Answer from the drawing. Dimensions are ordinates in mm from the lowest x, y and z of the part. Give positions to 0.01 mm unless a question says otherwise; leave off trailing zeros. Order: outer loops, then holes, each group sorted by start corner. A loop starts at its lowest first (then second) coordinate and runs counter-clockwise, first axis right, second up.
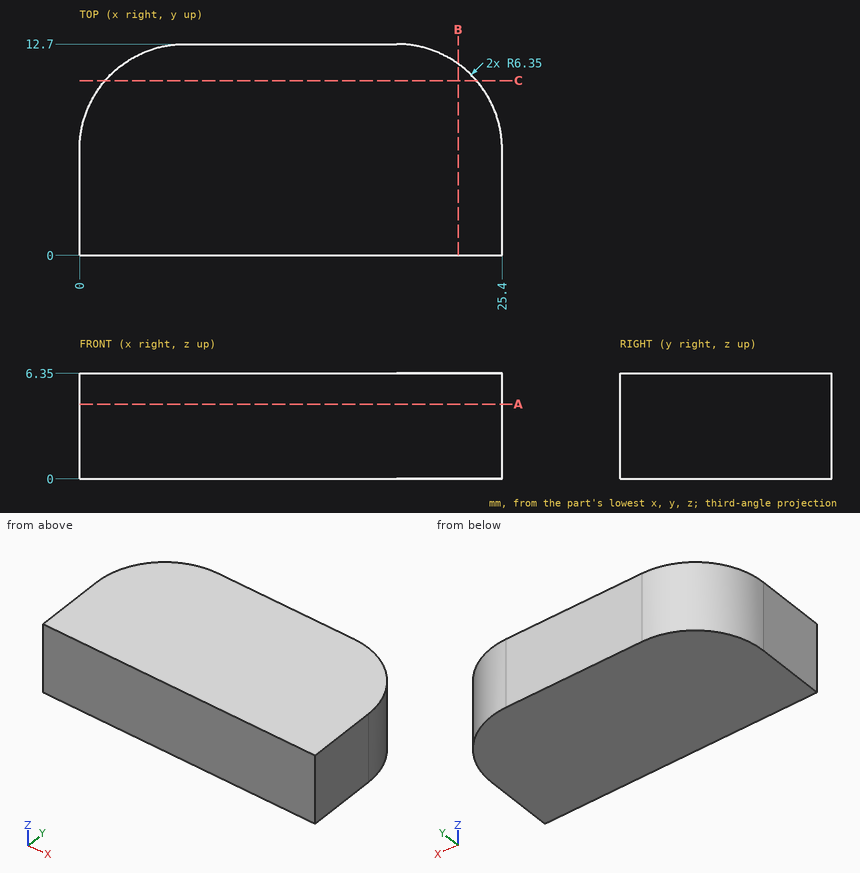
1. The part is cut by section B-B (x = 22.75). Write down the section's boundary in (y, z).
Findings below:
outline: (0, 0) - (11.51, 0) - (11.51, 6.35) - (0, 6.35) - close
2. The part is cut by section C-C (y = 10.5). Write down the section's boundary in (x, z).
Findings below:
outline: (1.54, 0) - (23.86, 0) - (23.86, 6.35) - (1.54, 6.35) - close
3. Straight lines are drawn through the part: probe 1 along Y at (x, z) = (20.25, 3.5); probe 2 along X at (y, z) = (6.75, 2.75); probe 3 along Y at (x, z) = (2.75, 2.75). For each, find the intervals that lie inside material, in ascending order.
Findings below:
probe 1: y = 0 to 12.59
probe 2: x = 0.01 to 25.39
probe 3: y = 0 to 11.58
4. The part is cut by section A-A (z = 4.5). Write down the section's boundary in (x, y), then the cut area to 3 significant figures.
Findings below:
outline: (0, 0) - (25.4, 0) - (25.4, 6.35) arc R6.35 ccw to (19.05, 12.7) - (6.35, 12.7) arc R6.35 ccw to (0, 6.35) - close
area: 305 mm2
